For this review, take the finished solid that the model builds, in its own axes (mm). Face numbers are marked on the shaded views. A direction names the side the tool comes from. Round coordinates to 2 decimals unless told otherwise and drop trailing zeros. Loops run counter-clockwise (first coordinate to the right, second up) from the corner with the lowest first, then second, coordinate; pieces in that order, holes last.
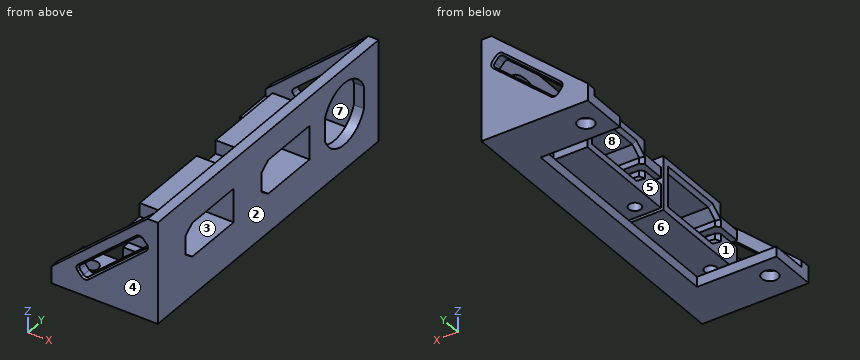
```python
from build123d import *

# Parameters (mm, degrees)
SKETCH4_R           = 2.4
BOSS_EXTRUDE4_DEPTH = 3
BOSS_EXTRUDE5_DEPTH = 30
CUT_EXTRUDE2_START  = -3
CUT_EXTRUDE2_DEPTH  = 148.103937837
SOCKETHOLES_DEPTH   = 3
CUT_EXTRUDE4_DEPTH  = 110
FILLET1_R           = 1
CHAMFER1_SIZE       = 0.5
SKETCH14_W          = 16
SKETCH14_H          = 32
BOSS_EXTRUDE6_DEPTH = 10
CUT_EXTRUDE5_DEPTH  = 10
CHAMFER2_SIZE       = 1
SKETCH18_R          = 1.8
CUT_EXTRUDE7_DEPTH  = 17
SKETCH19_R          = 1.8
CUT_EXTRUDE8_DEPTH  = 4


with BuildPart() as part:
    # Sketch4 → Boss-Extrude4 (new body)
    with BuildSketch(Plane.XY):
        Polygon((130.57, 0), (125.57, 0), (125.57, -34), (102.07, -34), (102.07, -45), (130.57, -45), align=None)
        with Locations((108.07, -40)):
            Circle(SKETCH4_R, mode=Mode.SUBTRACT)
    boss_extrude4 = extrude(amount=BOSS_EXTRUDE4_DEPTH)

    # Sketch4<10> → Boss-Extrude5 (add)
    with BuildSketch(Plane.XY):
        Polygon((133.57, 0), (130.57, 0), (130.57, -45), (102.07, -45), (102.07, -48), (121.666903009, -48), (133.57, -48), align=None)
    boss_extrude5 = extrude(amount=BOSS_EXTRUDE5_DEPTH)

    # Sketch11 → Cut-Extrude2 (cut)
    with BuildSketch(Plane(origin=(0, -45, 0), x_dir=(1, 0, 0), z_dir=(0, 1, 0)).offset(CUT_EXTRUDE2_START)):
        Polygon((102.07, -30), (130.57, -30), (102.07, -5), align=None)
    cut_extrude2 = extrude(amount=CUT_EXTRUDE2_DEPTH, mode=Mode.SUBTRACT)

    # Mirror2: Boss-Extrude4, Boss-Extrude5, Cut-Extrude2 across plane
    add(boss_extrude4.mirror(Plane.ZX))
    add(boss_extrude5.mirror(Plane.ZX))
    add(cut_extrude2.mirror(Plane.ZX), mode=Mode.SUBTRACT)

    # Socket holes → socketholes (cut)
    with BuildSketch(Plane.ZY.offset(-130.57)):
        Polygon((21.5, -33), (21.5, -15), (11.5, -15), (11.5, -33), (13.75, -36), (19.25, -36), align=None)
        with BuildLine():
            Line((19.749615362, 41.6), (13.250384638, 41.6))
            ThreePointArc((13.250384638, 41.6), (7.4, 33.1), (13.250384638, 24.6))
            Line((13.250384638, 24.6), (19.749615362, 24.6))
            ThreePointArc((19.749615362, 24.6), (23.996048952, 27.940615337), (25.6, 33.1))
            ThreePointArc((25.6, 33.1), (23.996048952, 38.259384663), (19.749615362, 41.6))
        make_face()
        Polygon((21.5, 18), (11.5, 18), (11.5, 0), (13.75, -3), (19.25, -3), (21.5, 0), align=None)
    extrude(amount=-SOCKETHOLES_DEPTH, mode=Mode.SUBTRACT)

    # Sketch12 → Cut-Extrude4 (cut)
    with BuildSketch(Plane.XZ.offset(48)):
        Polygon((109.618848481, 7.631156895), (128.261967636, 23.984770189), (130.57, 21.353613294), (111.926880845, 5), align=None)
    extrude(amount=-CUT_EXTRUDE4_DEPTH, mode=Mode.SUBTRACT)

    # Fillet1
    fillet1_edges = [part.edges().sort_by_distance(p)[0] for p in [
        (111.926880845, 46.5, 5),
        (109.618848481, 46.5, 7.631156895),
        (128.261967636, 46.5, 23.984770189),
        (130.57, 46.5, 21.353613294),
        (111.926880845, -46.5, 5),
        (109.618848481, -46.5, 7.631156895),
        (128.261967636, -46.5, 23.984770189),
        (130.57, -46.5, 21.353613294),
    ]]
    fillet(fillet1_edges, radius=FILLET1_R)

    # Chamfer1
    chamfer1_edges = [part.edges().sort_by_distance(p)[0] for p in [
        (110.772864663, 48, 6.315578448),
        (118.940408059, 48, 15.807963542),
        (121.248440423, 48, 13.176806647),
        (129.415983818, 48, 22.669191741),
        (121.248440423, -48, 13.176806647),
        (110.772864663, -48, 6.315578448),
        (118.940408059, -48, 15.807963542),
        (129.415983818, -48, 22.669191741),
        (110.032178493, 48, 7.604116614),
        (111.953921127, 48, 5.413330012),
        (130.156669988, 48, 21.380653575),
        (128.234927355, 48, 23.571440177),
        (111.953921127, -48, 5.413330012),
        (110.032178493, -48, 7.604116614),
        (128.234927355, -48, 23.571440177),
        (130.156669988, -48, 21.380653575),
    ]]
    chamfer(chamfer1_edges, length=CHAMFER1_SIZE)

    # Sketch14 → Boss-Extrude6 (add)
    # profile 1 of 2: a face of its own
    with BuildSketch(Plane.ZY.offset(-130.57)):
        Polygon((8.5, 21), (8.5, -1), (8.5, -11), (24.5, -11), (24.5, -1), (24.5, 21), align=None)
        Polygon((11.5, 0), (11.5, 18), (21.5, 18), (21.5, 0), (19.25, -3), (13.75, -3), align=None, mode=Mode.SUBTRACT)
    # profile 2 of 2: a face of its own
    with BuildSketch(Plane.ZY.offset(-130.57)):
        with Locations((16.5, -28)):
            Rectangle(SKETCH14_W, SKETCH14_H)
        Polygon((21.5, -33), (19.25, -36), (13.75, -36), (11.5, -33), (11.5, -15), (21.5, -15), align=None, mode=Mode.SUBTRACT)
    extrude(amount=BOSS_EXTRUDE6_DEPTH)

    # Sketch15 → Cut-Extrude5 (cut)
    with BuildSketch(Plane.ZY.offset(-120.57)):
        with BuildLine():
            Line((17.5, -36), (17.5, -44))
            ThreePointArc((17.5, -44), (16.5, -45), (15.5, -44))
            Line((15.5, -44), (15.5, -36))
            ThreePointArc((15.5, -36), (16.5, -35), (17.5, -36))
        make_face()
        with BuildLine():
            Line((15.5, -10.714079148), (15.5, -2.714079148))
            ThreePointArc((15.5, -2.714079148), (16.5, -1.714079148), (17.5, -2.714079148))
            Line((17.5, -2.714079148), (17.5, -10.714079148))
            ThreePointArc((17.5, -10.714079148), (16.5, -11.714079148), (15.5, -10.714079148))
        make_face()
    extrude(amount=-CUT_EXTRUDE5_DEPTH, mode=Mode.SUBTRACT)

    # Chamfer2
    chamfer2_edges = [part.edges().sort_by_distance(p)[0] for p in [
        (120.57, -34.5, 12.625),
        (120.57, -24, 11.5),
        (120.57, -15, 16.5),
        (120.57, -24, 21.5),
        (120.57, -34.5, 20.375),
        (120.57, -36, 18.375),
        (120.57, 9, 21.5),
        (120.57, 18, 16.5),
        (120.57, 9, 11.5),
        (120.57, -1.5, 12.625),
        (120.57, -3, 14.625),
        (120.57, -1.5, 20.375),
        (120.57, -3, 18.375),
        (120.57, -36, 14.625),
    ]]
    chamfer(chamfer2_edges, length=CHAMFER2_SIZE)

    # Sketch18 → Cut-Extrude7 (cut)
    with BuildSketch(Plane.XY.offset(24.5)):
        with Locations((125.57, -40)):
            Circle(SKETCH18_R)
        with Locations((125.57, -7)):
            Circle(SKETCH18_R)
    extrude(amount=-CUT_EXTRUDE7_DEPTH, mode=Mode.SUBTRACT)

    # Sketch19 → Cut-Extrude8 (cut)
    # profile 1 of 2: a face of its own
    with BuildSketch(Plane.XY.offset(24.5)):
        with BuildLine():
            Line((128.82, -44), (128.82, -40))
            ThreePointArc((128.82, -40), (127.868097039, -37.701902961), (125.57, -36.75))
            Line((125.57, -36.75), (120.57, -36.75))
            Line((120.57, -36.75), (120.57, -44))
            Line((120.57, -44), (128.82, -44))
        make_face()
        with Locations((125.57, -40)):
            Circle(SKETCH19_R, mode=Mode.SUBTRACT)
    # profile 2 of 2: a face of its own
    with BuildSketch(Plane.XY.offset(24.5)):
        with BuildLine():
            ThreePointArc((128.82, -7), (127.868097039, -4.701902961), (125.57, -3.75))
            Line((125.57, -3.75), (120.57, -3.75))
            Line((120.57, -3.75), (120.57, -11))
            Line((120.57, -11), (128.82, -11))
            Line((128.82, -11), (128.82, -7))
        make_face()
        with Locations((125.57, -7)):
            Circle(SKETCH19_R, mode=Mode.SUBTRACT)
    extrude(amount=-CUT_EXTRUDE8_DEPTH, mode=Mode.SUBTRACT)


solid = part.part
```
(1) Add section A-A (y = 10). Give the boundary of the cut face in (x, z).
(2) For L1, parallel to Z at x = 129, y = 13; L2, parallel to Y at x = 125.57, z = 18.75; L3, parallel to Y at x = 132, z = 14.75, list the stretches that pass through material, from the lowest coordinate up.
(3) Add section D-D (x = 118.5). Give the boundary of the cut face in (y, z).
(4) For the marked faces 5, 6, 7 and 8, list the 3-axis set-ups (+Z, -Z, +X, -X, +Y, -Y) from which the entire face can be reached by the end or side of a thin tool; tool diameter is ignored.
(5) Add section B-B (x = 108.07). Give the boundary of the cut face in (y, z), plus the area to 3 significant figures.
(6) Add section C-C (y = 40). Give the boundary of the cut face in (x, z), plus the area to 3 significant figures.
(7) Insertion check: pin 1 Ø3 at (x, y) = (125.57, -7) entering from +Z; pin 2 Ø13.5 at (y, z) = (15, 11.5) entering from -X; pin 3 Ø5 at (y, z) = (0.5, 18.5) entering from -X; pin 4 Ø8 at (x, y) = (126, 0.5) entering from +Z. Each pin has a flat end and moves straight along its axis. Give the tip position at first contact, or say it passes through.
(8) The part is to be moulded in two halves that separate along Y. For the marked faces 1, 2, 3 and 4, say which applies: pulls with the +Y half, pulls with the -Y half, needs draft (parallel to the pull), parting line crosses it, or undercut.
Outcome:
1. outline: (120.57, 8.5) - (130.57, 8.5) - (130.57, 3) - (125.57, 3) - (125.57, 0) - (133.57, 0) - (133.57, 11.5) - (121.57, 11.5) - (120.57, 10.5) - close; (120.57, 22.5) - (121.57, 21.5) - (133.57, 21.5) - (133.57, 30) - (130.57, 30) - (130.57, 24.5) - (120.57, 24.5) - close
2. L1: z = 0 to 3, 8.5 to 11.5, 21.5 to 24.5
2. L2: y = -44 to -41.8, -38.2 to -36, -15 to -12, -11 to -8.8, -5.2 to -3, 18 to 21
2. L3: y = -48 to -36, -15 to -3, 18 to 24.6, 41.6 to 48
3. outline: (-48, 0) - (-34, 0) - (-34, 3) - (-45, 3) - (-45, 10.77) - (-47.5, 10.77) - (-48, 10.1) - close; (-48, 16.09) - (-47.5, 15.42) - (-45, 15.42) - (-45, 19.41) - (-48, 19.41) - close; (34, 0) - (48, 0) - (48, 10.1) - (47.5, 10.77) - (45, 10.77) - (45, 3) - (34, 3) - close; (45, 15.42) - (47.5, 15.42) - (48, 16.09) - (48, 19.41) - (45, 19.41) - close
4. face 5: +Z, -Z, -X
4. face 6: -X
4. face 7: +Z, -X
4. face 8: +X, -X
5. outline: (-48, 0) - (-42.4, 0) - (-42.4, 3) - (-45, 3) - (-45, 10.26) - (-48, 10.26) - close; (-37.6, 0) - (-34, 0) - (-34, 3) - (-37.6, 3) - close; (34, 0) - (37.6, 0) - (37.6, 3) - (34, 3) - close; (42.4, 0) - (48, 0) - (48, 10.26) - (45, 10.26) - (45, 3) - (42.4, 3) - close
5. area: 98.8 mm2
6. outline: (102.07, 0) - (105.67, 0) - (105.67, 3) - (102.07, 3) - close; (110.47, 0) - (133.57, 0) - (133.57, 10.57) - (130.57, 10.57) - (130.57, 3) - (110.47, 3) - close; (130.57, 22.43) - (133.57, 22.43) - (133.57, 30) - (130.57, 30) - close
6. area: 126 mm2
7. pin 1: stops at z = 3
7. pin 2: stops at x = 120.57
7. pin 3: passes through
7. pin 4: stops at z = 24.5
8. face 1: undercut
8. face 2: needs draft
8. face 3: undercut
8. face 4: pulls with the -Y half
